```python
from build123d import *

# Parameters (mm, degrees)
F2_DEPTH = 25.4
F3_W     = 22.86
F3_H     = 25.4
F4_DEPTH = 2.54


with BuildPart() as f2:
    # F1 (on face) → F2 (new body)
    with BuildSketch(Plane.XZ):
        Polygon((-16.708008, 12.7), (-24.927931, 31.408676), (0, 31.408676), (0, 31.74649), (-37.627931, 31.74649), (-38.1, 0), (0, 0), (0, 12.7), align=None)
    extrude(amount=F2_DEPTH)

    # F3 (on face) → F4 (cut)
    with BuildSketch(Plane.XY.offset(31.74649)):
        with Locations((-11.43, -12.7)):
            Rectangle(F3_W, F3_H)
    extrude(amount=-F4_DEPTH, mode=Mode.SUBTRACT)


solid = f2.part
```
Could you check a few things on this model? Use its own coordinates, in mm. A direction names the side the tool comes from. Coordinates: 2 decimals unless noted, no trailing zeros. Write each loop counter-clockwise with the first axis right and the second up, starting at its lowest first coordinate (ties: lowest second). Pieces come first, ordered by that corner, then holes. Notation, with made-up numbers: (7.5, -27.5) -> (39.5, -27.5) arc R18 cw to (39.5, -12.5) -> close; hole circle Ø6 at (20.5, -17). An arc over 180 degrees is marked (long way). One line per question, with ' | ' between items. Start each with the question number.
1. For faces 1 (the face through (-24, 0, 13)), 2 (the face through (-24, -13, 31.409)), which set-ups out of +Z, -Z, +X, -X, +Y, -Y let a thin tool reach every point of the face, with its end or its side?
2. Please list where these lines run through material, in increasing order: line 1 along Z through (x, y) = (-11, -15); line 2 along X through (y, z) = (-9.75, 26.5); line 3 along X through (y, z) = (-17.5, 18).
3. If we section it at A-A (y = -9): Please give me the cut outline in (x, z).
4. Will these pins go through, and if not, where does the flat tip stop? P1, Ø8.5, axis at x = -7.5, y = -12.5, coming from the +Z side; P2, Ø1.5, axis at y = -9, z = 10, coming from the -X side; P3, Ø1, axis at y = -22, z = 21.5, coming from the +X side.
5. If we section it at C-C (z = 24.5): Please give me the cut outline in (x, y), and give its area (3 significant figures).
6. If we section it at B-B (x = -11): Please give me the cut outline in (y, z), and give its area (3 significant figures).
7. Thinking about a two-plate mould opening in Z: for faces 3 (the face through (-19, -13, 0)), 4 (the face through (-8, -13, 12.7)), 5 (the face through (-20.76, -12.52, 21.92)), which applies, pulls with the +Z half, pulls with the -Z half, needs draft (parallel to the pull), parting line crosses it, or undercut?
Return value:
1) face 1: +Z, -Z, +X, -X, +Y | face 2: +X, +Y, -Y
2) line 1: z = 0 to 12.7 | line 2: x = -37.71 to -22.77 | line 3: x = -37.83 to -19.04
3) outline: (-38.1, 0) -> (0, 0) -> (0, 12.7) -> (-16.71, 12.7) -> (-24.93, 31.41) -> (-22.86, 31.41) -> (-22.86, 31.75) -> (-37.63, 31.75) -> close
4) P1: stops at z = 12.7 | P2: stops at x = -37.96 | P3: stops at x = -20.35
5) outline: (-37.74, -25.4) -> (-21.89, -25.4) -> (-21.89, 0) -> (-37.74, 0) -> close | area: 402 mm²
6) outline: (-25.4, 0) -> (0, 0) -> (0, 12.7) -> (-25.4, 12.7) -> close | area: 323 mm²
7) face 3: pulls with the -Z half | face 4: pulls with the +Z half | face 5: undercut
